```python
from build123d import *

# Parameters (mm, degrees)
SMUSSO1_SIZE                = 3
SMUSSO2_SIZE                = 1
RIPETIZIONECIRCOLARE1_COUNT = 6
FORO_FILETTATO_M4_1_D       = 3.3
RIPETIZIONECIRCOLARE2_COUNT = 12


with BuildPart() as part:
    # Schizzo1 → Rivoluzione1 (revolve)
    with BuildSketch(Plane.XY, mode=Mode.PRIVATE) as rivoluzione1_sk:
        Polygon((72.5, 31.559405291), (72.5, 5.559405291), (31.5, 5.559405291), (31.5, 12.559405291), (54.5, 12.559405291), (54.5, 31.559405291), align=None)
    revolve(rivoluzione1_sk.sketch.rotate(Axis((0, 82.574074074, 0), (0, -1, 0)), 90), axis=Axis((0, 82.574074074, 0), (0, -1, 0)))

    # Smusso1
    smusso1_edges = [part.edges().sort_by_distance(p)[0] for p in [
        (0, 5.559405291, -72.5),
    ]]
    chamfer(smusso1_edges, length=SMUSSO1_SIZE)

    # Smusso2
    smusso2_edges = [part.edges().sort_by_distance(p)[0] for p in [
        (0, 12.559405291, -31.5),
        (0, 5.559405291, -31.5),
    ]]
    chamfer(smusso2_edges, length=SMUSSO2_SIZE)

    # Schizzo3 → Foro filettato M8-1 (revolve, cut)
    with BuildSketch(Plane(origin=(0, 31.559405291, -62), x_dir=(0, 0, 1), z_dir=(1, 0, 0))):
        Polygon((0, 0), (0, 21.042926105), (3.4, 19), (3.4, 0), align=None)
    foro_filettato_m8_1 = revolve(axis=Axis((0, 37.909405291, -62), (0, -1, 0)), mode=Mode.SUBTRACT)

    # RipetizioneCircolare1: Foro filettato M8-1 ×6 about axis
    ripetizionecircolare1_axis = Axis((0, 0, 0), (0, 1, 0))
    for i in range(1, RIPETIZIONECIRCOLARE1_COUNT):
        add(foro_filettato_m8_1.rotate(ripetizionecircolare1_axis, i * 360 / RIPETIZIONECIRCOLARE1_COUNT), mode=Mode.SUBTRACT)

    # Foro filettato M4-1 (through all)
    with Locations(Plane(origin=(0, 12.559405291, 0), x_dir=(1, 0, 0), z_dir=(0, 1, 0))):
        with Locations((0, 46), (0, 37.5)):
            foro_filettato_m4_1 = Hole(FORO_FILETTATO_M4_1_D / 2)

    # RipetizioneCircolare2: Foro filettato M4-1 ×12 about axis
    ripetizionecircolare2_axis = Axis((0, 0, 0), (0, 1, 0))
    for i in range(1, RIPETIZIONECIRCOLARE2_COUNT):
        add(foro_filettato_m4_1.rotate(ripetizionecircolare2_axis, i * 360 / RIPETIZIONECIRCOLARE2_COUNT), mode=Mode.SUBTRACT)


solid = part.part
```
Build history of the part. All positions in model axes, mm. A direction names the side the tool comes from. Coordinates: 2 decimals unless noted, no trailing zeros. Order: outer loops, then holes, each group sorted by start corner. A loop starts at its lowest first (then second) coordinate and runs counter-clockwise, first axis right, second up. Notation, with made-up numbers: (55, 1.5) -> (102, 1.5) arc R21 ccw to (102, 15.5) -> close; hole circle Ø4 at (29.5, 41.5). An arc over 180 degrees is marked (long way). Answer in a Markdown table with one row per item. Add a question column.
Q1. Which spindle directions (+Z, -Z, +X, -X, +Y, -Y) get a long thin tool onto all of the face, cutting with end or side? Do faces 1 (the face through (-1.021, 22.192, -58.757)), 2 (the face through (-41.486, 9.01, -22.927)). Say none if no direction does.
Q2. Wall check: line 1 along Z through (x, y) = (-1, 28.5); line 2 along X through (y, z) = (12, -24.5); line 3 along Y through (x, z) = (-16, -46). Give the ranges that are in metal, low to high. Write a range as [from, to].
Q3. Drop flat-ended pins along their axis: pin 1 (8 mm diameter, centred on x = 21.5, y = 12.5, fed in from -Z); pin 2 (5.5 mm diameter, centred on x = -32.48, z = 18.75, fed in from +Y); pin 3 (8 mm diameter, centred on y = 16.5, z = 58, fed in from +X); pin 4 (2.5 mm diameter, centred on x = 32.48, z = 18.75, fed in from +Y). Give the stop position or say it passes through.
Q4. Band-saw the part on A-A, the plane y = 18.5. List the corners of the cut face in (x, z), then the cut area to 3 significant figures.
Q5. Mould opens along X. For faces 3 (the face through (0.89, 9.01, 47.39)), 4 (the face through (14, 5.559, 30)) say: +X half, -X half, draft (parallel to the pull), parting line (faces both ways), or undercut.
Answers follow:
| question | item | result |
|---|---|---|
| 1 | face 1 | +Y |
| 1 | face 2 | +Y, -Y |
| 2 | line 1 | [-72.49, -65.25], [-58.75, -54.49], [54.49, 58.75], [65.25, 72.49] |
| 2 | line 2 | [-68.23, -40.52], [-39.15, -20.49], [20.49, 39.15], [40.52, 68.23] |
| 2 | line 3 | [5.56, 12.56] |
| 3 | pin 1 | z = -70.36 |
| 3 | pin 2 | y = 12.56 |
| 3 | pin 3 | x = 48.38 |
| 3 | pin 4 | through |
| 4 | outline | circle Ø145 at (0, 0); hole circle Ø6.8 at (-53.69, -31); hole circle Ø6.8 at (-53.69, 31); hole circle Ø109 at (0, 0); hole circle Ø6.8 at (0, -62); hole circle Ø6.8 at (0, 62); hole circle Ø6.8 at (53.69, -31); hole circle Ø6.8 at (53.69, 31) |
| 4 | area | 6,960 mm^2 |
| 5 | face 3 | undercut |
| 5 | face 4 | draft |
